Input: part model. Units: mm. Frame: model coordinates. A direction names the side the tool comes from. Round coordinates to 2 decimals unless told otherwise and drop trailing zeros. Loops run counter-clockwise (first coordinate to the right, second up) from the corner with the lowest first, then second, coordinate; pieces in that order, holes last. Notation, with made-up numbers: (71, 51) -> (80, 51) arc R33 ccw to (80, 84) -> close; hole circle Ø4 at (20, 49.5). An arc over 180 degrees is marked (long way). Answer in a Markdown table with one row per item. Add a question column.
Q1. Section B-B, the plane y = 2.05. Output: boundary loops of the cut face in (x, z), and give its area (3 significant figures).
Q2. Ray query, L1, parallel to X at y = 2.35, z = -6; L2, parallel to Z at x = 28, y = 3.8; L3, parallel to Z at x = 37, y = 3.8. Return the intervals inside material, ascending. Write a range as from..to.
Q3. Section A-A, the plane z = -6. Output: boundary loops of the cut face in (x, y), and give its area (3 significant figures).
Q4. Pin query (flat end, axial travel): pin 1 (2.5 mm diameter, centred on y = 3.5, z = 3.5, fed in from +X). Return the tip coordinate at first contact, or that it passes through.
Q5. Section D-D, the plane z = -35. Output: boundary loops of the cut face in (x, y).
Q6. Reachability of faces 1 (the face through (15, 2, 3)), 2 (the face through (35, 2, -12)), 3 (the face through (20.594, 2, -47)), 4 (the face through (12, 2, -45)), 5 (the face through (35.946, 2.465, -55.037)) from +Z, -Z, +X, -X, +Y, -Y: full face, straight path, thin tool, end or side. Return the list, or none.
Q7. Section C-C, the plane x = 9. Output: boundary loops of the cut face in (y, z).
Q8. Mould query, pull axis Z, two halves, no side actions, for faces 6 (the face through (30, 2, 0)), 7 (the face through (40.305, 2.465, -66.345)), 8 (the face through (19, 5, -32)). Classes: pulls with the +Z half, pulls with the -Z half, needs draft (parallel to the pull), parting line crosses it, or undercut.
```python
from build123d import *

# Parameters (mm, degrees)
SKETCH2_R           = 14
SKETCH2_R_2         = 2
SKETCH2_R_3         = 0.7
SKETCH2_W           = 5
SKETCH2_H           = 5
SKETCH2_R_4         = 3
SKETCH2_W_2         = 15
BOSS_EXTRUDE2_DEPTH = 5


with BuildPart() as part:
    # Sketch2 → Boss-Extrude2 (new body)
    # profile 1 of 6: a face of its own
    with BuildSketch(Plane(origin=(0, 0, 0), x_dir=(1, 0, 0), z_dir=(0, 1, 0))):
        with Locations((34.59438676, 53.562546918)):
            Circle(SKETCH2_R)
        with Locations(Location((34.59438676, 53.562546918, 0), (0, 0, 270))):
            Circle(SKETCH2_R_2, mode=Mode.SUBTRACT)
        with Locations(Location((34.557412927, 42.562609058, 0), (0, 0, 270))):
            Circle(SKETCH2_R_3, mode=Mode.SUBTRACT)
        with Locations(Location((25.086648049, 59.094536127, 0), (0, 0, 270))):
            Circle(SKETCH2_R_3, mode=Mode.SUBTRACT)
        with Locations(Location((44.139099303, 59.03049557, 0), (0, 0, 270))):
            Circle(SKETCH2_R_3, mode=Mode.SUBTRACT)
    # profile 2 of 6: a face of its own
    with BuildSketch(Plane(origin=(0, 0, 0), x_dir=(1, 0, 0), z_dir=(0, 1, 0))):
        with BuildLine():
            ThreePointArc((44.493881696, 43.663051982), (29.236818707, 40.628233463), (20.59438676, 53.562546918))
            Line((20.59438676, 53.562546918), (20.59438676, 40))
            Line((20.59438676, 40), (23.964739417, 40))
            Line((23.964739417, 40), (23.964739417, 23.133909702))
            Line((23.964739417, 23.133909702), (27.177730802, 26.346901087))
            Line((27.177730802, 26.346901087), (44.493881696, 43.663051982))
        make_face()
    # profile 3 of 6: a face of its own
    with BuildSketch(Plane(origin=(0, 0, 0), x_dir=(1, 0, 0), z_dir=(0, 1, 0))):
        Polygon((23.964739417, 40), (20.59438676, 40), (15, 40), (10, 40), (0, 40), (0, 0), (15, 0), (23.964739417, 0), (23.964739417, 12), (23.964739417, 23.133909702), align=None)
    # profile 4 of 6: a face of its own
    with BuildSketch(Plane(origin=(0, 0, 0), x_dir=(1, 0, 0), z_dir=(0, 1, 0))):
        with Locations((12.5, 42.5)):
            Rectangle(SKETCH2_W, SKETCH2_H)
    # profile 5 of 6: a face of its own
    with BuildSketch(Plane(origin=(0, 0, 0), x_dir=(1, 0, 0), z_dir=(0, 1, 0))):
        with BuildLine():
            Line((45, 12), (23.964739417, 12))
            Line((23.964739417, 12), (23.964739417, 0))
            Line((23.964739417, 0), (45, 0))
            ThreePointArc((45, 0), (51, 6), (45, 12))
        make_face()
        with Locations(Location((45, 6, 0), (0, 0, 270))):
            Circle(SKETCH2_R_4, mode=Mode.SUBTRACT)
    # profile 6 of 6: a face of its own
    with BuildSketch(Plane(origin=(0, 0, 0), x_dir=(1, 0, 0), z_dir=(0, 1, 0))):
        with Locations((7.5, -2.5)):
            Rectangle(SKETCH2_W_2, SKETCH2_H)
    extrude(amount=BOSS_EXTRUDE2_DEPTH)


solid = part.part
```
Answer block:
| question | item | result |
|---|---|---|
| 1 | outline | (0, -40) -> (10, -40) -> (10, -45) -> (15, -45) -> (15, -40) -> (20.59, -40) -> (20.59, -53.56) arc R14 ccw (long way) to (44.49, -43.66) -> (23.96, -23.13) -> (23.96, -12) -> (45, -12) arc R6 ccw to (45, 0) -> (15, 0) -> (15, 5) -> (0, 5) -> close; hole circle Ø1.4 at (25.09, -59.09); hole circle Ø4 at (34.59, -53.56); hole circle Ø1.4 at (34.56, -42.56); hole circle Ø6 at (45, -6); hole circle Ø1.4 at (44.14, -59.03) |
| 1 | area | 2,120 mm^2 |
| 2 | L1 | 0..42, 48..51 |
| 2 | L2 | -65.91..-27.17, -12..0 |
| 2 | L3 | -67.35..-36.17, -12..0 |
| 3 | outline | (0, 0) -> (42, 0) -> (42, 5) -> (0, 5) -> close; (48, 0) -> (51, 0) -> (51, 5) -> (48, 5) -> close |
| 3 | area | 225 mm^2 |
| 4 | pin 1 | x = 15 |
| 5 | outline | (0, 0) -> (35.83, 0) -> (35.83, 5) -> (0, 5) -> close |
| 6 | face 1 | +Z, +X, +Y, -Y |
| 6 | face 2 | +X, +Y, -Y |
| 6 | face 3 | -Z, +Y, -Y |
| 6 | face 4 | -Z, -X, +Y, -Y |
| 6 | face 5 | +Y, -Y |
| 7 | outline | (0, -40) -> (5, -40) -> (5, 5) -> (0, 5) -> close |
| 8 | face 6 | pulls with the +Z half |
| 8 | face 7 | undercut |
| 8 | face 8 | needs draft |
